Can you work these out from the model? Positions are in its coordinate system, mm. A direction names the side the tool comes from. Give positions to 0.01 mm unless a question says otherwise; leave off trailing zeros. Order: outer loops, then holes, each group sorted by start corner. A loop starts at its lowest first (then second) coordinate and runs counter-clockwise, first axis right, second up.
```python
from build123d import *

# Parameters (mm, degrees)
F1_DEPTH = 50
F2_W     = 25
F2_H     = 15
F3_DEPTH = 10.001
F4_W     = 25
F4_H     = 15
F5_DEPTH = 10.001


with BuildPart() as f1:
    # F0 (on Right) → F1 (new body)
    with BuildSketch(Plane.YZ):
        Polygon((0, 10), (0, 0), (30, 0), (30, 30), (20, 30), (20, 10), align=None)
    extrude(amount=F1_DEPTH)

    # F2 (on face) → F3 (cut, through all)
    with BuildSketch(Plane.XZ.offset(-20)):
        with Locations((12.5, 22.5)):
            Rectangle(F2_W, F2_H)
    extrude(amount=-F3_DEPTH, mode=Mode.SUBTRACT)

    # F4 (on face) → F5 (cut, through all)
    with BuildSketch(Plane.XY.offset(10)):
        with Locations((37.5, 7.5)):
            Rectangle(F4_W, F4_H)
    extrude(amount=-F5_DEPTH, mode=Mode.SUBTRACT)


solid = f1.part
```
1) Suppose I cut it at A-A (x = 14.5). Please give me the cut outline in (y, z), and give its area (3 significant figures).
2) Suppose I cut it at C-C (y = 18). Please give me the cut outline in (x, z).
3) I'm going to push flat-ended pins straight in: pin 1 Ø12 at (y, z) = (5.5, 11.5) entering from +X; pin 2 Ø1 at (x, z) = (16.5, 12) entering from -Y; pin 3 Ø3 at (y, z) = (22.5, 21) entering from -X; pin 4 Ø5 at (x, y) = (28, 17.5) entering from -Z. Where does each tip first touch, or does it pass through?
4) Suppose I cut it at B-B (z = 9.25). Please give me the cut outline in (x, y), and give its area (4 significant figures).
5) Suppose I cut it at D-D (y = 4). Please give me the cut outline in (x, z), and give its area (3 significant figures).
6) Which directions (+Z, -Z, +X, -X, +Y, -Y) give clear straight access to the entire face, cutting with the end or side of a thin tool? Please do faces 1 (the face through (19, 18, 0)), 2 (the face through (36, 20, 18)), 3 (the face through (25, 7, 5)), 4 (the face through (30, 30, 11)), 5 (the face through (12, 25, 15)).
7) If I drill on line 1 (Z direction, x = 8.5, y = 8); line 2 (X direction, y = 23.75, z = 23); line 3 (Y direction, x = 26, z = 6.5), over which ranges is the centre line in solid material (lowest first)?
Results:
1. outline: (0, 0) - (30, 0) - (30, 15) - (20, 15) - (20, 10) - (0, 10) - close
1. area: 350 mm2
2. outline: (0, 0) - (50, 0) - (50, 10) - (0, 10) - close
3. pin 1: stops at x = 25
3. pin 2: stops at y = 20
3. pin 3: stops at x = 25
3. pin 4: stops at z = 0
4. outline: (0, 0) - (25, 0) - (25, 15) - (50, 15) - (50, 30) - (0, 30) - close
4. area: 1,125 mm2
5. outline: (0, 0) - (25, 0) - (25, 10) - (0, 10) - close
5. area: 250 mm2
6. face 1: -Z, +X, -X, +Y, -Y
6. face 2: +Z, +X, -X, -Y
6. face 3: +Z, -Z, +X, -Y
6. face 4: +Z, -Z, +X, -X, +Y
6. face 5: +Z, -X, +Y, -Y
7. line 1: z = 0 to 10
7. line 2: x = 25 to 50
7. line 3: y = 15 to 30
